Geometry: final body of the model. Coordinates: model frame, mm. A direction names the side the tool comes from. Coordinates: 2 decimals unless noted, no trailing zeros. Write each loop counter-clockwise with the first axis right and the second up, starting at its lowest first coordinate (ties: lowest second). Pieces come first, ordered by that corner, then holes. Notation, with made-up numbers: M 71,-13 L 127,-13 A7 ccw 127,-8 Z; hole C -11,-2.5 d3. An arc over 180 degrees is marked long. Write item = value, one per line. Start each with the question number.
Item 1: Section B-B on z = 0. Output: boundary loops of the cut face in (x, y).
Item 2: First-contact query: pin 1 Ø2 at (x, z) = (22.5, 41) entering from +Y; pin 2 Ø12 at (y, z) = (-97.5, 0) entering from +X. Flat tips, straight axial feed; report the tip coordinate or a pass-through.
Item 3: Pull-direction query (Y, two-part tool) for faces 1 (the flat face through (20.05, -2, 1)), 2 (the flat face through (69, -5, 1)), 3 (the flat face through (-30, 0, -1)); classes: +Y half, -Y half, draft (parallel to the pull), parting line (faces both ways), or undercut.
Item 4: Reachability of faces 4 (the flat face through (-2, -48, -87.5)), 5 (the flat face through (-20.05, -2, 1)), 6 (the flat face through (-2, -46, -82.5)), 7 (the flat face through (-2, -125, -1)), 8 (the flat face through (1, -97, -85)) from +Z, -Z, +X, -X, +Y, -Y: full face, straight path, thin tool, end or side. Return the list, or none.
Item 5: Section C-C on y = -16. Output: boundary loops of the cut face in (x, z).
Item 6: Section A-A on x = -0.5. Output: boundary loops of the cut face in (y, z).
Item 7: Ray query, L1, parallel to X at y = -109, z = 8; L2, parallel to Y at x = 122.45, z = 0; L3, parallel to Z at x = -62.5, y = -96.5. Return the intervals inside material, ascending. Write a range as [from, to].
Item 8: Section D-D on x = -63. Output: boundary loops of the cut face in (y, z), plus the area to 4 significant figures.
from build123d import *

# Parameters (mm, degrees)
SKETCH1_W           = 250
SKETCH1_H           = 175
BOSS_EXTRUDE1_DEPTH = 125
SKETCH2_W           = 240
SKETCH2_H           = 165
CUT_EXTRUDE1_DEPTH  = 120
SKETCH3_W           = 40.1
SKETCH3_H           = 165
CUT_EXTRUDE2_DEPTH  = 126
SKETCH4_R           = 7.5
CUT_EXTRUDE3_DEPTH  = 251
SKETCH6_W           = 250
SKETCH6_H           = 175
BOSS_EXTRUDE2_DEPTH = 5
SKETCH7_W           = 200
SKETCH7_H           = 23
CUT_EXTRUDE4_DEPTH  = 5


with BuildPart() as part:
    # Sketch1 → Boss-Extrude1 (new body)
    with BuildSketch(Plane(origin=(0, 0, 0), x_dir=(1, 0, 0), z_dir=(0, 1, 0))):
        Rectangle(SKETCH1_W, SKETCH1_H)
    extrude(amount=-BOSS_EXTRUDE1_DEPTH)

    # Sketch2 → Cut-Extrude1 (cut)
    with BuildSketch(Plane.XZ.offset(125)):
        Rectangle(SKETCH2_W, SKETCH2_H)
    extrude(amount=-CUT_EXTRUDE1_DEPTH, mode=Mode.SUBTRACT)

    # Sketch3 → Cut-Extrude2 (cut, through all)
    with BuildSketch(Plane(origin=(0, 0, 0), x_dir=(1, 0, 0), z_dir=(0, 1, 0))):
        Rectangle(SKETCH3_W, SKETCH3_H)
    extrude(amount=-CUT_EXTRUDE2_DEPTH, mode=Mode.SUBTRACT)

    # Sketch4 → Cut-Extrude3 (cut, through all)
    with BuildSketch(Plane.ZY.offset(125)):
        with Locations((0, -97.5)):
            Circle(SKETCH4_R)
    extrude(amount=-CUT_EXTRUDE3_DEPTH, mode=Mode.SUBTRACT)

    # Sketch6 → Boss-Extrude2 (add)
    with BuildSketch(Plane.XZ.offset(125)):
        Rectangle(SKETCH6_W, SKETCH6_H)
    extrude(amount=-BOSS_EXTRUDE2_DEPTH)

    # Sketch7 → Cut-Extrude4 (cut)
    with BuildSketch(Plane(origin=(0, 0, -87.5), x_dir=(-1, 0, 0), z_dir=(0, 0, -1))):
        with Locations((0, -108.5)):
            Rectangle(SKETCH7_W, SKETCH7_H)
    extrude(amount=-CUT_EXTRUDE4_DEPTH, mode=Mode.SUBTRACT)


solid = part.part
Responses:
q1.outline = M -125,-125 L 125,-125 L 125,-105 L 120,-105 L 120,-120 L -120,-120 L -120,-105 L -125,-105 Z; M -125,-90 L -120,-90 L -120,-5 L -20.05,-5 L -20.05,0 L -125,0 Z; M 20.05,-5 L 120,-5 L 120,-90 L 125,-90 L 125,0 L 20.05,0 Z
q2.pin_1 = 0
q2.pin_2 = through
q3.face_1 = draft
q3.face_2 = undercut
q3.face_3 = +Y half
q4.face_4 = -Z, +X, -X, +Y, -Y
q4.face_5 = +Y
q4.face_6 = none
q4.face_7 = +Z, -Z, +X, -X, -Y
q4.face_8 = -Z
q5.outline = M -125,-87.5 L 125,-87.5 L 125,87.5 L -125,87.5 Z; hole M -120,-82.5 L 120,-82.5 L 120,82.5 L -120,82.5 Z
q6.outline = M -125,-87.5 L -120,-87.5 L -120,82.5 L 0,82.5 L 0,87.5 L -125,87.5 Z; M -97,-87.5 L 0,-87.5 L 0,-82.5 L -97,-82.5 Z
q7.L1 = [-125, -120], [120, 125]
q7.L2 = [-125, -105], [-90, 0]
q7.L3 = [-87.5, -82.5], [82.5, 87.5]
q8.outline = M -125,-87.5 L -120,-87.5 L -120,82.5 L -5,82.5 L -5,-82.5 L -97,-82.5 L -97,-87.5 L 0,-87.5 L 0,87.5 L -125,87.5 Z
q8.area = 2,785 mm²
